Work out the finished part from the listing and answer in its coordinate system (mm). A direction names the side the tool comes from. Coordinates: 2 decimals unless noted, no trailing zeros. Order: outer loops, then holes, each group sorted by start corner. A loop starts at its lowest first (then second) coordinate and runs counter-clockwise, first axis right, second up. Notation, with made-up numbers: (38, 17.5) -> (44, 17.5) arc R12 ccw to (44, 27.5) -> close; hole circle Ø5 at (19.25, 14). An arc over 180 degrees is marked (long way). Write item = value, one per line. Start each with the question number.
Q1. The part is cut by section A-A, the plane x = 0. Determine the outline of the cut face in (y, z) (3 decimals), plus the area to 3 significant figures.
Q2. A flat-ended cylindrical pin translates along its axis: pin 1 (1 mm diameter, centred on y = -1, z = -3.5, fed in from +X). Find the tip coordinate at first contact, or state that the pin passes through.
Q3. The part is cut by section B-B, the plane z = -2.25. Determine the outline of the cut face in (x, y).
Q4. Which of the six approach directions +Z, -Z, +X, -X, +Y, -Y give full straight-line access (tool end or side, diameter ignored) to faces 1 (the flat face through (0, -1, 1.5)), 2 (the cylindrical face through (0, -1, -3)), 3 (the flat face through (0, -0.75, 1))?
Q5. Straight lines are drawn through the part: L1, parallel to X at y = -0.5, z = -2; L2, parallel to Z at x = 1.3, y = -1.05. For each, find the intervals that lie inside material, in ascending order. Write a range as from..to.
```python
from build123d import *

# Parameters (mm, degrees)
F_0135_CYLINDER_SKETCH_R    = 2.5
F_0135_CYLINDER_DEPTH       = 1.5
F_0136_FILLET_R             = 0.375
F_0137_EXTRUDE_DEPTH        = 0.835
F_0137_EXTRUDE_ROTATE_ANGLE = 120
F_0140_CYLINDER_SKETCH_R    = 1
F_0140_CYLINDER_DEPTH       = 5.7
F_0141_CONE_ROTATE_ANGLE    = 90


with BuildPart() as part:
    # 0135_cylinder_Sketch → 0135_cylinder (new body)
    with BuildSketch(Plane.XY):
        Circle(F_0135_CYLINDER_SKETCH_R)
    extrude(amount=F_0135_CYLINDER_DEPTH)

    # 0136_fillet
    f_0136_fillet_edges = [part.edges().sort_by_distance(p)[0] for p in [
        (-2.5, 0, 1.5),
    ]]
    fillet(f_0136_fillet_edges, radius=F_0136_FILLET_R)


with BuildPart() as body_2:
    # 0137_extrude_Sketch → 0137_extrude (new body)
    with BuildSketch(Plane.XY):
        Polygon((0, 0), (0.866025404, 0), (1.299038106, 0.75), (0.866025404, 1.5), (0, 1.5), (-0.433012702, 0.75), align=None)
    extrude(amount=F_0137_EXTRUDE_DEPTH)


with BuildPart() as body_2_1:
    # 0137_extrude_Rotate: read off the stored shape, not the designer's step
    # 0137_extrude_Rotate: moved
    add(body_2.part.rotate(Axis((0, 0, 0), (0, 0, 1)), F_0137_EXTRUDE_ROTATE_ANGLE))


with BuildPart() as body_2_2:
    # 0137_extrude_Translate: moved
    add(body_2_1.part.moved(Location((0.866025404, 0, 0.675))))


with BuildPart() as part_1:
    add(part.part)

    # 0139_sub: cut body 2
    add(body_2_2.part, mode=Mode.SUBTRACT)


with BuildPart() as body_2_2_1:
    # 0140_cylinder_Sketch → 0140_cylinder (new body)
    with BuildSketch(Plane.XY):
        Circle(F_0140_CYLINDER_SKETCH_R)
    extrude(amount=F_0140_CYLINDER_DEPTH)


with BuildPart() as body_2_2_2:
    # 0140_cylinder_Translate: moved
    add(body_2_2_1.part.moved(Location((0, 0, -5.7))))


with BuildPart() as body_3:
    # 0141_cone_Sketch → 0141_cone (revolve)
    with BuildSketch(Plane.XY, mode=Mode.PRIVATE) as f_0141_cone_sk:
        Polygon((0, 0), (1, 0), (0.7, 0.3), (0, 0.3), align=None)
    revolve(f_0141_cone_sk.sketch.rotate(Axis((0, -100, 0), (0, 1, 0)), 90), axis=Axis((0, -100, 0), (0, 1, 0)))


with BuildPart() as body_3_1:
    # 0141_cone_Rotate: moved
    add(body_3.part.rotate(Axis((0, 0, 0), (1, 0, 0)), F_0141_CONE_ROTATE_ANGLE))


with BuildPart() as body_3_2:
    # 0141_cone_Translate: moved
    add(body_3_1.part.moved(Location((0, 0, -6))))


with BuildPart() as body_2_2_3:
    add(body_2_2_2.part)

    # 0143_add: union body 3
    add(body_3_2.part)


with BuildPart() as part_2:
    add(part_1.part)

    # 0144_add: union body 2 2
    add(body_2_2_3.part)


solid = part_2.part
```
Model answer:
q1.outline = (-2.5, 0) -> (-1, 0) -> (-1, -5.7) -> (-0.7, -5.7) -> (-1, -6) -> (1, -6) -> (0.7, -5.7) -> (1, -5.7) -> (1, 0) -> (2.5, 0) -> (2.5, 1.125) arc R0.375 ccw to (2.125, 1.5) -> (0.75, 1.5) -> (0.75, 0.675) -> (-0.75, 0.675) -> (-0.75, 1.5) -> (-2.125, 1.5) arc R0.375 ccw to (-2.5, 1.125) -> close
q1.area = 18.1 mm2
q2.pin_1 = 0.87
q3.outline = circle Ø2 at (0, 0)
q4.face_1 = +Z, +X, -X, +Y, -Y
q4.face_2 = -Z
q4.face_3 = +Z
q5.L1 = -0.87..0.87
q5.L2 = 0..1.5
